Input: dimensioned drawing with shaded views. Units: mm. Origin: part minimum x, y, z. A direction names the side the tool comes from. Coordinates: 2 decimals unless noted, no trailing zeros. Order: outer loops, then holes, each group sorted by start corner. A loop starts at its lowest first (then second) coordinate and runs counter-clockwise, first axis right, second up. Notation, with made-up numbers: (51, -19.75) -> (57, -19.75) arc R9 cw to (57, -7.75) -> close; hole circle Ø8 at (88.5, -39). An arc over 180 degrees is marked (long way). Answer as CSV lines item,"result".
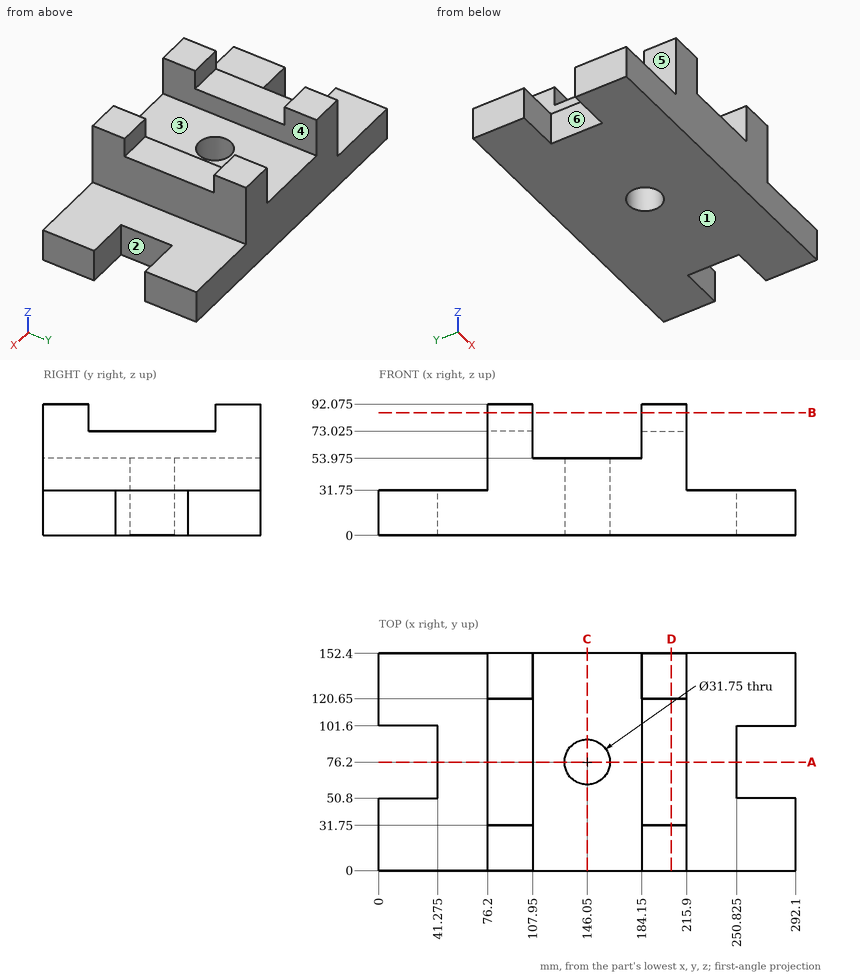
1. Cut plane B-B (z = 86). Return the cut outline in (x, y), plus the area to 3 significant figures.
Findings:
outline,"(76.2, 0) -> (107.95, 0) -> (107.95, 31.75) -> (76.2, 31.75) -> close; (76.2, 120.65) -> (107.95, 120.65) -> (107.95, 152.4) -> (76.2, 152.4) -> close; (184.15, 0) -> (215.9, 0) -> (215.9, 31.75) -> (184.15, 31.75) -> close; (184.15, 120.65) -> (215.9, 120.65) -> (215.9, 152.4) -> (184.15, 152.4) -> close"
area,"4,030 mm2"
2. Cut plane C-C (x = 146.05). Return the cut outline in (y, z) (3 decimals), plus the area to 3 significant figures.
Findings:
outline,"(0, 0) -> (60.325, 0) -> (60.325, 53.975) -> (0, 53.975) -> close; (92.075, 0) -> (152.4, 0) -> (152.4, 53.975) -> (92.075, 53.975) -> close"
area,"6,510 mm2"
3. Reachability of the marked faces 4, 5 and 6 from +Z, -Z, +X, -X, +Y, -Y: full face, straight path, thin tool, end or side. Return the list, or none.
Findings:
face 4,"+Z, +Y, -Y"
face 5,"+Z, -X, +Y, -Y"
face 6,"+Z, -Z, -X"
4. Cut plane A-A (y = 76.2). Return the cut outline in (x, z) (3 decimals).
Findings:
outline,"(41.275, 0) -> (130.175, 0) -> (130.175, 53.975) -> (107.95, 53.975) -> (107.95, 73.025) -> (76.2, 73.025) -> (76.2, 31.75) -> (41.275, 31.75) -> close; (161.925, 0) -> (250.825, 0) -> (250.825, 31.75) -> (215.9, 31.75) -> (215.9, 73.025) -> (184.15, 73.025) -> (184.15, 53.975) -> (161.925, 53.975) -> close"
5. Ray query, line 1 along Y through (x, z) = (41, 25); line 2 along X through (y, z) = (76.2, 20.5) (3 decimals); line 3 along X through (y, z) = (76, 33). Return the intervals inside material, ascending.
Findings:
line 1,"y = 0 to 50.8, 101.6 to 152.4"
line 2,"x = 41.275 to 130.175, 161.925 to 250.825"
line 3,"x = 76.2 to 130.18, 161.92 to 215.9"
6. Contact query for flat-ended pins moving along their axis: pin 1 (16 mm diameter, centred on y = 73.5, z = 17, fed in from +X) (3 decimals); pin 2 (23 mm diameter, centred on x = 137.5, y = 101, fed in from +Z) (3 decimals); pin 3 (4 mm diameter, centred on x = 251, y = 80, fed in from +Z). Output: stop coordinate, or through.
Findings:
pin 1,"stops at x = 250.825"
pin 2,"stops at z = 53.975"
pin 3,"stops at z = 31.75"
7. Mould query, pull axis X, two halves, no side actions, for the marked faces 1, 2 and 3. Classes: released by +X, released by -X, zero draft, split by the parting line, or undercut.
Findings:
face 1,"zero draft"
face 2,"released by +X"
face 3,"undercut"
8. Cut plane D-D (x = 205). Return the cut outline in (y, z) (3 decimals), plus the area to 3 significant figures.
Findings:
outline,"(0, 0) -> (152.4, 0) -> (152.4, 92.075) -> (120.65, 92.075) -> (120.65, 73.025) -> (31.75, 73.025) -> (31.75, 92.075) -> (0, 92.075) -> close"
area,"12,300 mm2"
